Verification items for the finished model (mm, model axes). Face numbers are marked on the shaded views. Give positions to 0.01 mm unless a question says otherwise; leave off trailing zeros. Order: outer loops, then holes, each group sorted by start corner. A loop starts at its lowest first (then second) coordinate and runs counter-clockwise, first axis right, second up. Notation, with made-up numbers: M 14.5,17 L 27.5,17 A20 ccw 27.5,29 Z; hole C -34.5,52.25 d4. An arc over 180 degrees is marked long. Answer as a JSON object with one key per item and string values.
```python
from build123d import *

# Parameters (mm, degrees)
EXTRUDE_1_DEPTH     = 30
SKETCH_2_R          = 2.1
CUT_EXTRUDE_1_DEPTH = 30
CUT_EXTRUDE_START   = -5
SKETCH_3_R          = 4
CUT_EXTRUDE_2_DEPTH = 8.5


with BuildPart() as part:
    # 草圖1 → 填料-伸長1 (new body)
    with BuildSketch(Plane.XY):
        Polygon((0, 0), (15, 0), (0, 12.5), align=None)
    extrude(amount=EXTRUDE_1_DEPTH)

    # 草圖2 → 除料-伸長1 (cut)
    with BuildSketch(Plane(origin=(0, 0, 0), x_dir=(-1, 0, 0), z_dir=(0, -1, 0))):
        with Locations((-7.5, -20.7)):
            Circle(SKETCH_2_R)
        with Locations((-7.5, -9.3)):
            Circle(SKETCH_2_R)
    extrude(amount=-CUT_EXTRUDE_1_DEPTH, mode=Mode.SUBTRACT)

    # 草圖3 → 除料-伸長2 (cut, through all)
    with BuildSketch(Plane.XZ.offset(CUT_EXTRUDE_START)):
        with Locations((7.5, 20.7)):
            Circle(SKETCH_3_R)
        with Locations((7.5, 9.3)):
            Circle(SKETCH_3_R)
    extrude(amount=-CUT_EXTRUDE_2_DEPTH, mode=Mode.SUBTRACT)


solid = part.part
```
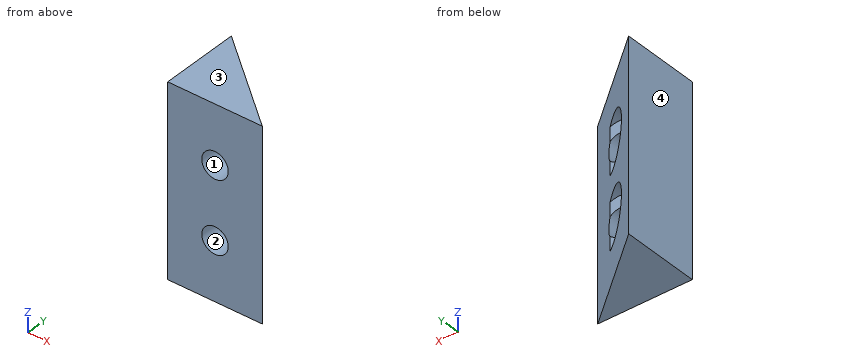
Q1. Release check for a two-part mould opening along X. For the marked faces 1, 2, 3 and 4 record: +X half, -X half, draft (parallel to the pull), parting line (faces both ways), or undercut.
Resolved:
{"face 1": "undercut", "face 2": "undercut", "face 3": "draft", "face 4": "-X half"}
Q2. Section check D-D on y = 9. Record the cut outline in (x, z), then the cut area to 3 significant figures.
Resolved:
{"outline": "M 0,0 L 4.2,0 L 4.2,7.04 A4 cw 4.2,11.56 L 4.2,18.44 A4 cw 4.2,22.96 L 4.2,30 L 0,30 Z", "area": "122 mm²"}
Q3. Section check A-A on z = 20.7. Record the cut outline in (x, y).
Resolved:
{"outline": "M 0,0 L 5.4,0 L 5.4,5 L 3.5,5 L 3.5,9.58 L 0,12.5 Z; M 9.6,0 L 15,0 L 9.6,4.5 Z"}
Q4. Section check C-C on y = 4.5. Record the cut outline in (x, z).
Resolved:
{"outline": "M 0,0 L 9.6,0 L 9.6,30 L 0,30 Z; hole C 7.5,9.3 d4.2; hole C 7.5,20.7 d4.2"}
Q5. Material ranges on L1, parallel to Z at x = 7.5, y = 6.15; L2, parallel to Z at x = 7.5, y = 3.2; L3, parallel to Y at x = 4.5, z = 11, recorded low to high.
Resolved:
{"L1": "z = 0 to 5.3, 13.3 to 16.7, 24.7 to 30", "L2": "z = 0 to 7.2, 11.4 to 18.6, 22.8 to 30", "L3": "y = 0 to 5"}
Q6. Gauge pin test, flat ends, axial feed: pin 1 Ø3 at (x, z) = (7.5, 19) entering from +Y; pin 2 Ø4 at (y, z) = (9, 22) entering from +X. Record the tip position at first contact, or that the pin passes through.
Resolved:
{"pin 1": "stops at y = 5", "pin 2": "stops at x = 5.06"}
Q7. Section check B-B on x = 7.5. Record the cut outline in (y, z).
Resolved:
{"outline": "M 0,0 L 6.25,0 L 6.25,5.3 L 5,5.3 L 5,7.2 L 0,7.2 Z; M 0,11.4 L 5,11.4 L 5,13.3 L 6.25,13.3 L 6.25,16.7 L 5,16.7 L 5,18.6 L 0,18.6 Z; M 0,22.8 L 5,22.8 L 5,24.7 L 6.25,24.7 L 6.25,30 L 0,30 Z"}
